Part model, mm, in its own coordinate system. Face numbers are marked on the shaded views. A direction names the side the tool comes from. Give positions to 0.01 mm unless a question says otherwise; leave off trailing zeros. Loops run counter-clockwise (first coordinate to the right, second up) from the corner with the lowest first, then second, coordinate; pieces in that order, holes last. Notation, with made-up numbers: M 76.5,43 L 106.5,43 A18 cw 106.5,59 Z; hole C 46.5,82.25 d2. An arc over 180 degrees is marked long. Answer in a Markdown table with one row per item.
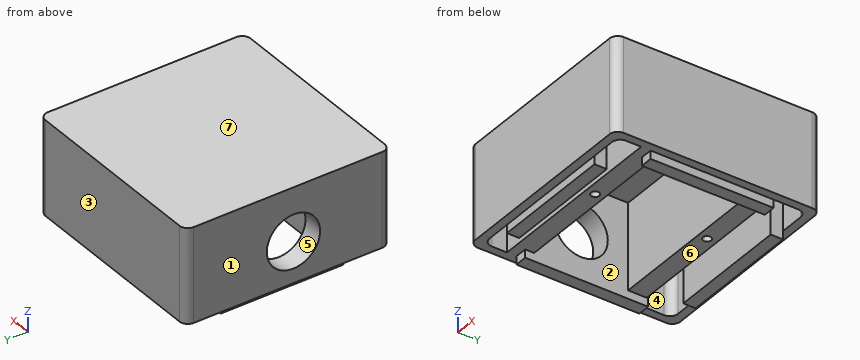
from build123d import *

# Parameters (mm, degrees)
SZKIC1_W                           = 30
SZKIC1_H                           = 3
DODANIE_WYCI_GNI_CIE1_DEPTH        = 23
DODANIE_WYCI_GNI_CIE1_DEPTH_BACK   = 2
SZKIC1_W_2                         = 3
SZKIC1_H_2                         = 30
DODANIE_WYCI_GNI_CIE1_2_DEPTH      = 23
DODANIE_WYCI_GNI_CIE1_2_DEPTH_BACK = 2
DODANIE_WYCI_GNI_CIE1_3_DEPTH      = 23
DODANIE_WYCI_GNI_CIE1_3_DEPTH_BACK = 2
DODANIE_WYCI_GNI_CIE1_4_DEPTH      = 23
DODANIE_WYCI_GNI_CIE1_4_DEPTH_BACK = 2
SZKIC2_W                           = 50
SZKIC2_H                           = 50
DODANIE_WYCI_GNI_CIE2_DEPTH        = 23
SZKIC3_W                           = 11.8
SZKIC3_H                           = 4.5
SZKIC3_R                           = 1
SZKIC3_W_2                         = 10.1
SZKIC3_W_3                         = 18.1
DODANIE_WYCI_GNI_CIE3_DEPTH        = 23
ZAOKR_GLENIE1_R                    = 2
WYTNIJ_WYCI_GNI_CIE1_REACH         = 52
SZKIC4_R                           = 6.5
SZKIC5_W                           = 46
SZKIC5_H                           = 46
DODANIE_WYCI_GNI_CIE4_DEPTH        = 2
DODANIE_WYCI_GNI_CIE5_START        = -10
SZKIC6_R                           = 1.05
SZKIC6_R_2                         = 1
DODANIE_WYCI_GNI_CIE5_DEPTH        = 11


with BuildPart() as part:
    # Szkic1 → Dodanie-wyci_gni_cie1 (new body, two sides)
    with BuildSketch(Plane.XY) as dodanie_wyci_gni_cie1_sk:
        with Locations((0, 21.5)):
            Rectangle(SZKIC1_W, SZKIC1_H)
    extrude(amount=DODANIE_WYCI_GNI_CIE1_DEPTH)
    extrude(dodanie_wyci_gni_cie1_sk.sketch, amount=-DODANIE_WYCI_GNI_CIE1_DEPTH_BACK)



with BuildPart() as body_2:
    # Szkic1 → Dodanie-wyci_gni_cie1 2 (new body, two sides)
    with BuildSketch(Plane.XY) as dodanie_wyci_gni_cie1_2_sk:
        with Locations((21.5, 0)):
            Rectangle(SZKIC1_W_2, SZKIC1_H_2)
    extrude(amount=DODANIE_WYCI_GNI_CIE1_2_DEPTH)
    extrude(dodanie_wyci_gni_cie1_2_sk.sketch, amount=-DODANIE_WYCI_GNI_CIE1_2_DEPTH_BACK)


with BuildPart() as body_3:
    # Szkic1 → Dodanie-wyci_gni_cie1 3 (new body, two sides)
    with BuildSketch(Plane.XY) as dodanie_wyci_gni_cie1_3_sk:
        with Locations((0, -21.5)):
            Rectangle(SZKIC1_W, SZKIC1_H)
    extrude(amount=DODANIE_WYCI_GNI_CIE1_3_DEPTH)
    extrude(dodanie_wyci_gni_cie1_3_sk.sketch, amount=-DODANIE_WYCI_GNI_CIE1_3_DEPTH_BACK)


with BuildPart() as body_4:
    # Szkic1 → Dodanie-wyci_gni_cie1 4 (new body, two sides)
    with BuildSketch(Plane.XY) as dodanie_wyci_gni_cie1_4_sk:
        with Locations((-21.5, 0)):
            Rectangle(SZKIC1_W_2, SZKIC1_H_2)
    extrude(amount=DODANIE_WYCI_GNI_CIE1_4_DEPTH)
    extrude(dodanie_wyci_gni_cie1_4_sk.sketch, amount=-DODANIE_WYCI_GNI_CIE1_4_DEPTH_BACK)


with BuildPart() as part_1:
    add(part.part)

    add(body_2.part)  # Dodanie-wyci_gni_cie2 merges body 2

    add(body_3.part)  # Dodanie-wyci_gni_cie2 merges body 3

    add(body_4.part)  # Dodanie-wyci_gni_cie2 merges body 4
    # Szkic2 → Dodanie-wyci_gni_cie2 (add)
    with BuildSketch(Plane.XY):
        Rectangle(SZKIC2_W, SZKIC2_H)
        with BuildLine():
            Line((-21, -23), (21, -23))
            ThreePointArc((21, -23), (22.414213562, -22.414213562), (23, -21))
            Line((23, -21), (23, 21))
            ThreePointArc((23, 21), (22.414213562, 22.414213562), (21, 23))
            Line((21, 23), (-21, 23))
            ThreePointArc((-21, 23), (-22.414213562, 22.414213562), (-23, 21))
            Line((-23, 21), (-23, -21))
            ThreePointArc((-23, -21), (-22.414213562, -22.414213562), (-21, -23))
        make_face(mode=Mode.SUBTRACT)
    extrude(amount=DODANIE_WYCI_GNI_CIE2_DEPTH)

    # Szkic3 → Dodanie-wyci_gni_cie3 (add)
    with BuildSketch(Plane.XY.offset(23)):
        Polygon((-1.9, -17.3), (-1.9, -12.8), (-20, -12.8), (-20, -15), (-23, -15), (-23, -17.3), align=None)
        with Locations((4, -15.05)):
            Rectangle(SZKIC3_W, SZKIC3_H)
        with Locations((4, -15)):
            Circle(SZKIC3_R, mode=Mode.SUBTRACT)
        Polygon((20, -12.8), (9.9, -12.8), (9.9, -17.3), (23, -17.3), (23, -15), (20, -15), align=None)
        with Locations((14.95, 12.35)):
            Rectangle(SZKIC3_W_2, SZKIC3_H)
        with Locations((4, 12.35)):
            Rectangle(SZKIC3_W, SZKIC3_H)
        with Locations((4, 12.3)):
            Circle(SZKIC3_R, mode=Mode.SUBTRACT)
        with Locations((-10.95, 12.35)):
            Rectangle(SZKIC3_W_3, SZKIC3_H)
    extrude(amount=-DODANIE_WYCI_GNI_CIE3_DEPTH)

    # Zaokr_glenie1
    zaokr_glenie1_edges = [part_1.edges().sort_by_distance(p)[0] for p in [
        (-25, -25, 11.5),
        (-25, 25, 11.5),
        (25, 25, 11.5),
        (25, -25, 11.5),
    ]]
    fillet(zaokr_glenie1_edges, radius=ZAOKR_GLENIE1_R)

    # Szkic4 → Wytnij-wyci_gni_cie1 (cut, up to next)
    with BuildSketch(Plane.ZY.offset(25), mode=Mode.PRIVATE) as wytnij_wyci_gni_cie1_sk1:
        with Locations((10, -1.35)):
            Circle(SZKIC4_R)
    wytnij_wyci_gni_cie1_tool1 = extrude(wytnij_wyci_gni_cie1_sk1.sketch, amount=-WYTNIJ_WYCI_GNI_CIE1_REACH, mode=Mode.PRIVATE) & part_1.part
    add(wytnij_wyci_gni_cie1_tool1.solids().sort_by_distance((-25, -1.35, 10))[0], mode=Mode.SUBTRACT)

    # Szkic5 → Dodanie-wyci_gni_cie4 (add)
    with BuildSketch(Plane.XY.offset(23)):
        Rectangle(SZKIC5_W, SZKIC5_H)
    extrude(amount=-DODANIE_WYCI_GNI_CIE4_DEPTH)

    # Szkic6 → Dodanie-wyci_gni_cie5 (add)
    with BuildSketch(Plane(origin=(0, 0, 0), x_dir=(-1, 0, 0), z_dir=(0, 0, -1)).offset(DODANIE_WYCI_GNI_CIE5_START)):
        with Locations((-4, 12.25)):
            Circle(SZKIC6_R)
        with Locations((-4, -15)):
            Circle(SZKIC6_R_2)
    extrude(amount=-DODANIE_WYCI_GNI_CIE5_DEPTH)


solid = part_1.part
(1) Saw through at C-C (z = 2). Give the number of separate pieces and of enclosed holes in the cut face, plus the area to 3 significant figures.
Recorded:
| item | result |
|---|---|
| separate pieces | 1 |
| enclosed holes | 5 |
| area | 1,110 mm^2 |
(2) Saw through at D-D (y = -2). Write the cut outline in (x, z).
Recorded:
| item | result |
|---|---|
| outline | M -25,0 L -23,0 L -23,-2 L -20,-2 L -20,3.53 L -25,3.53 Z; M -25,16.47 L -20,16.47 L -20,21 L 20,21 L 20,-2 L 23,-2 L 23,0 L 25,0 L 25,23 L -25,23 Z |
(3) Pin check, flat tips, straight feed: pin 1 Ø1.5 at (x, y) = (-5.5, 17.5) entering from -Z; pin 2 Ø0.6 at (x, y) = (4, 12) entering from -Z; pin 3 Ø5 at (y, z) = (-3, 5.5) entering from -X; pin 4 Ø1.5 at (x, y) = (-17.5, 11.5) entering from -Z. Stop position of each tip, or through.
Recorded:
| item | result |
|---|---|
| pin 1 | stops at z = 21 |
| pin 2 | stops at z = 10 |
| pin 3 | stops at x = -25 |
| pin 4 | stops at z = 0 |
(4) Drill centre lines: line 1 along Y through (x, z) = (4, 3.5); line 2 along Y through (x, z) = (4.5, 12.25); line 3 along X through (y, z) = (-10, 3.25). Where is each one in solid material? Low to high.
Recorded:
| item | result |
|---|---|
| line 1 | y = -25 to -20, -17.3 to -16, -14 to -12.8, 10.1 to 11.3, 13.3 to 14.6, 20 to 25 |
| line 2 | y = -25 to -20, -17.3 to -12.8, 10.1 to 14.6, 20 to 25 |
| line 3 | x = -25 to -20, 20 to 25 |
(5) Which spindle directions (+Z, -Z, +X, -X, +Y, -Y) get a long thin tool onto all of the face, cutting with end or side? Do the marked faces 5, 6 and 7. Say none if no direction does.
Recorded:
| item | result |
|---|---|
| face 5 | -X |
| face 6 | -Z |
| face 7 | +Z, +X, -X, +Y, -Y |
(6) Saw through at B-B (y = 12.3). Write the cut outline in (x, z), plus the area to 3 significant figures.
Recorded:
| item | result |
|---|---|
| outline | M -25,0 L -23,0 L -23,-2 L -20,-2 L -20,0 L 3,0 L 3,10 L 5,10 L 5,0 L 20,0 L 20,-2 L 23,-2 L 23,0 L 25,0 L 25,23 L -25,23 Z |
| area | 1,140 mm^2 |
(7) Saw through at A-A (x = -2.5). Write the cut outline in (y, z), plus the area to 3 significant figures.
Recorded:
| item | result |
|---|---|
| outline | M -25,0 L -23,0 L -23,-2 L -20,-2 L -20,21 L -17.3,21 L -17.3,0 L -12.8,0 L -12.8,21 L 10.1,21 L 10.1,0 L 14.6,0 L 14.6,21 L 20,21 L 20,-2 L 23,-2 L 23,0 L 25,0 L 25,23 L -25,23 Z |
| area | 511 mm^2 |
(8) Pull direction X, two halves, no side cores. Call the marked faces 1, 2, 3 and 4: +X half, -X half, draft (parallel to the pull), parting line (faces both ways), or undercut.
Recorded:
| item | result |
|---|---|
| face 1 | -X half |
| face 2 | undercut |
| face 3 | draft |
| face 4 | undercut |
